from build123d import *

# Parameters (mm, degrees)
BOSS_EXTRUDE1_DEPTH = 5
SKETCH2_R           = 20
CUT_EXTRUDE1_DEPTH  = 6
SKETCH3_R           = 30
CUT_EXTRUDE2_DEPTH  = 2
SKETCH4_R           = 2.5
SKETCH4_R_2         = 19.05
CUT_EXTRUDE3_DEPTH  = 6


with BuildPart() as part:
    # Sketch1 → Boss-Extrude1 (new body)
    with BuildSketch(Plane(origin=(0, 0, 0), x_dir=(1, 0, 0), z_dir=(0, 1, 0))):
        with BuildLine():
            ThreePointArc((-100, 53), (-153, 0), (-100, -53))
            Line((-100, -53), (-100, 53))
        make_face()
        with BuildLine():
            Line((-100, 53), (-100, -53))
            ThreePointArc((-100, -53), (-62.523340597, -37.476659403), (-47, 0))
            ThreePointArc((-47, 0), (-62.523340597, 37.476659403), (-100, 53))
        make_face()
        with BuildLine():
            ThreePointArc((-47, 0), (-62.523340597, -37.476659403), (-100, -53))
            Line((-100, -53), (100, -53))
            ThreePointArc((100, -53), (47, 0), (100, 53))
            Line((100, 53), (-100, 53))
            ThreePointArc((-100, 53), (-62.523340597, 37.476659403), (-47, 0))
        make_face()
        with BuildLine():
            ThreePointArc((100, 53), (47, 0), (100, -53))
            Line((100, -53), (100, 53))
        make_face()
        with BuildLine():
            Line((100, 53), (100, -53))
            ThreePointArc((100, -53), (137.476659403, -37.476659403), (153, 0))
            ThreePointArc((153, 0), (137.476659403, 37.476659403), (100, 53))
        make_face()
    extrude(amount=BOSS_EXTRUDE1_DEPTH)

    # Sketch2 → Cut-Extrude1 (cut, through all)
    with BuildSketch(Plane(origin=(0, 5, 0), x_dir=(1, 0, 0), z_dir=(0, 1, 0))):
        with Locations((100, 0)):
            Circle(SKETCH2_R)
    extrude(amount=-CUT_EXTRUDE1_DEPTH, mode=Mode.SUBTRACT)

    # Sketch3 → Cut-Extrude2 (cut)
    with BuildSketch(Plane.XZ):
        with Locations((100, 0)):
            Circle(SKETCH3_R)
    extrude(amount=-CUT_EXTRUDE2_DEPTH, mode=Mode.SUBTRACT)

    # Sketch4 → Cut-Extrude3 (cut, through all)
    with BuildSketch(Plane(origin=(0, 5, 0), x_dir=(1, 0, 0), z_dir=(0, 1, 0))):
        with Locations((-123.57, 23.57)):
            Circle(SKETCH4_R)
        with Locations((-76.43, 23.57)):
            Circle(SKETCH4_R)
        with Locations((-76.43, -23.57)):
            Circle(SKETCH4_R)
        with Locations((-123.57, -23.57)):
            Circle(SKETCH4_R)
        with Locations((-100, 0)):
            Circle(SKETCH4_R_2)
        with BuildLine():
            Line((45.182638641, 10), (45.182638641, 30))
            ThreePointArc((45.182638641, 30), (42.682638641, 32.5), (40.182638641, 30))
            Line((40.182638641, 30), (40.182638641, 10))
            ThreePointArc((40.182638641, 10), (42.682638641, 7.5), (45.182638641, 10))
        make_face()
        with BuildLine():
            Line((40.182638641, -10), (40.182638641, -30))
            ThreePointArc((40.182638641, -30), (42.682638641, -32.5), (45.182638641, -30))
            Line((45.182638641, -30), (45.182638641, -10))
            ThreePointArc((45.182638641, -10), (42.682638641, -7.5), (40.182638641, -10))
        make_face()
    extrude(amount=-CUT_EXTRUDE3_DEPTH, mode=Mode.SUBTRACT)


solid = part.part
Part model, mm, in its own coordinate system. A direction names the side the tool comes from. Give positions to 0.01 mm unless a question says otherwise; leave off trailing zeros. Write each loop counter-clockwise with the first axis right and the second up, starting at its lowest first coordinate (ties: lowest second). Pieces come first, ordered by that corner, then holes.
1) Which spindle directions (+Z, -Z, +X, -X, +Y, -Y) get a long thin tool onto all of the face, cutting with end or side? Do faces 5 (the face through (70.03, 0.99, 1.32)), 6 (the face through (-2, 0, -1)), 7 (the face through (40.183, 3, -20)). Say none if no direction does.
Resolved:
face 5: -Y
face 6: +Z, -Z, +X, -X, -Y
face 7: +Y, -Y
2) Pin check, flat tips, straight feed: pin 1 (6.5 mm diameter, centred on x = -76.43, z = 23.57, fed in from -Y); pin 2 (3 mm diameter, centred on y = 3, z = -39.5, fed in from -X); pin 3 (4 mm diameter, centred on x = -76.43, z = -23.57, fed in from +Y); pin 4 (1 mm diameter, centred on y = 2, z = -37, fed in from +X). Stop position of each tip, or through.
Resolved:
pin 1: stops at y = 0
pin 2: stops at x = -136.95
pin 3: passes through
pin 4: stops at x = 138.43
3) Cut at C-C on z = -42. Write the cut outline in (x, y).
Resolved:
outline: (-132.33, 0) - (132.33, 0) - (132.33, 5) - (-132.33, 5) - close
4) Two-plate mould, pull along X, no slides. Class faces 1 (the face through (-78.928, 2.535, 23.46)), 2 (the face through (-152.987, 2.465, -1.165)), 3 (the face through (80.02, 3.52, -0.88)), 4 (the face through (1, 2, -53)): released by +X, released by -X, zero draft, split by the parting line, or undercut.
Resolved:
face 1: undercut
face 2: released by -X
face 3: undercut
face 4: zero draft
5) Cut at B-B on x = -112.5. Write the cut outline in (y, z), then the cut area to 3 significant figures.
Resolved:
outline: (0, -51.5) - (5, -51.5) - (5, -14.38) - (0, -14.38) - close; (0, 14.38) - (5, 14.38) - (5, 51.5) - (0, 51.5) - close
area: 371 mm2
6) Probe L1, parallel to Z at x = -76.43, y = 2.1; L2, parallel to X at y = 0.35, z = -8; L3, parallel to X at y = 2.65, z = 13.5. List the from-to ranges inside material, lowest first.
Resolved:
L1: z = -53 to -26.07, -21.07 to 21.07, 26.07 to 53
L2: x = -152.39 to -117.29, -82.71 to 41.18, 44.18 to 71.09, 128.91 to 152.39
L3: x = -151.25 to -113.44, -86.56 to 40.18, 45.18 to 85.24, 114.76 to 151.25
7) Cut at A-A on y = 0.95. State how many separate pieces and enclosed holes the cut face has, then the cut area to 3 significant figures.
Resolved:
separate pieces: 1
enclosed holes: 8
area: 25,700 mm2
